```python
from build123d import *

# Parameters (mm, degrees)
SKETCH1_W                   = 58
SKETCH1_H                   = 13
BOSS_EXTRUDE1_DEPTH         = 30
FILLET1_R                   = 2
FILLET2_R                   = 3
M6_TAPPED_HOLE1_D           = 5
M6_TAPPED_HOLE1_DEPTH       = 17
M6_TAPPED_HOLE1_CSINK_D     = 6.05
M6_TAPPED_HOLE1_CSINK_ANGLE = 90
M6_TAPPED_HOLE1_TIP         = 1.502151548
CUT_EXTRUDE1_DEPTH          = 24


with BuildPart() as part:
    # Sketch1 → Boss-Extrude1 (new body)
    with BuildSketch(Plane(origin=(0, 0, 0), x_dir=(1, 0, 0), z_dir=(0, 1, 0))):
        Rectangle(SKETCH1_W, SKETCH1_H)
    extrude(amount=-BOSS_EXTRUDE1_DEPTH)

    # Fillet1
    fillet1_edges = [part.edges().sort_by_distance(p)[0] for p in [
        (29, -15, 6.5),
        (-29, -15, 6.5),
        (-29, -15, -6.5),
        (29, -15, -6.5),
    ]]
    fillet(fillet1_edges, radius=FILLET1_R)

    # Fillet2
    # the kernel refuses this fillet: 3 mm, written as the material it takes off along each edge
    with BuildSketch(Plane(origin=(-34.5, 0, 6.5), x_dir=(0, -1, 0), z_dir=(1, 0, 0))) as fillet2_piece_1:
        with BuildLine():
            CenterArc((FILLET2_R, FILLET2_R), FILLET2_R, 180, 90)
            Line((0, FILLET2_R), (0, 0))
            Line((0, 0), (FILLET2_R, 0))
        make_face()
    extrude(amount=69, mode=Mode.SUBTRACT)

    # M6 Tapped Hole1
    with Locations(Plane(origin=(0, -30, 0), x_dir=(-1, 0, 0), z_dir=(0, -1, 0))):
        with Locations((-21.5, 0), (21.5, 0)):
            CounterSinkHole(M6_TAPPED_HOLE1_D / 2, M6_TAPPED_HOLE1_CSINK_D / 2, depth=M6_TAPPED_HOLE1_DEPTH, counter_sink_angle=M6_TAPPED_HOLE1_CSINK_ANGLE)
            with Locations((0, 0, -(M6_TAPPED_HOLE1_DEPTH + M6_TAPPED_HOLE1_TIP / 2))):  # 118° drill point
                Cone(0, M6_TAPPED_HOLE1_D / 2, M6_TAPPED_HOLE1_TIP, mode=Mode.SUBTRACT)

    # Sketch5 → Cut-Extrude1 (cut, symmetric)
    with BuildSketch(Plane(origin=(0, 0, 0), x_dir=(0, 0, -1), z_dir=(1, 0, 0))):
        Polygon((-6.5, -8), (-6.115988572, -30), (-6.5, -30), align=None)
    extrude(amount=CUT_EXTRUDE1_DEPTH, both=True, mode=Mode.SUBTRACT)


solid = part.part
```
CAD build for the part. Positions are in the model's coordinates, mm. A direction names the side the tool comes from. Give positions to 0.01 mm unless a question says otherwise; leave off trailing zeros. Order: outer loops, then holes, each group sorted by start corner. A loop starts at its lowest first (then second) coordinate and runs counter-clockwise, first axis right, second up. Notation, with made-up numbers: M 57.5,34.5 L 66.5,34.5 A32 ccw 66.5,73.5 Z; hole C 83,20.25 d1. An arc over 180 degrees is marked long. Put each result on its own line as item: value. Start each with the question number.
(1) Drill centre lines: line 1 along X through (y, z) = (-29, 1.5); line 2 along X through (y, z) = (-25, 0.5); line 3 along Z through (x, y) = (21.5, -21.5). Where is each one in solid material? Low to high.
(2) Saw through at B-B, the plane x = 4.5. Write the cut outline in (y, z), then the cut area to 3 significant figures.
(3) Saw through at A-A, the plane y = -27.5. Write the cut outline in (x, z), then the cut area to 3 significant figures.
(4) Saw through at C-C, the plane y = -19. Write the cut outline in (x, z).
(5) Flat gauge pin, fed straight in: pin 1 Ø6.5 at (x, z) = (-21.5, 0) entering from +Y. Where does the tip first touch, or does it go through?
(6) Which spindle directions (+Z, -Z, +X, -X, +Y, -Y) get a long thin tool onto all of the face, cutting with end or side? Do faces 1 (the cylindrical face through (19, -21, 0)), 2 (the flat face through (29, -15, 0)). Say none if no direction does.
(7) Mould opens along Z. For faces 3 (the flat face through (0, 0, -2)), 4 (the flat face through (-2, -6, 6.5)), 5 (the cylindrical face through (-24, -21, 0)) say: +Z half, -Z half, draft (parallel to the pull), parting line (faces both ways), or undercut.
Check result:
1. line 1: x = -29 to -23.5, -19.5 to 19.5, 23.5 to 29
1. line 2: x = -29 to -23.95, -19.05 to 19.05, 23.95 to 29
1. line 3: z = -6.5 to -2.5, 2.5 to 6.26
2. outline: M -30,-6.5 L 0,-6.5 L 0,3.5 A3 ccw -3,6.5 L -8,6.5 L -30,6.12 Z
2. area: 384 mm2
3. outline: M -29,-4.5 A2 ccw -27,-6.5 L 27,-6.5 A2 ccw 29,-4.5 L 29,4.5 A2 ccw 27,6.5 L 24,6.5 L 24,6.16 L -24,6.16 L -24,6.5 L -27,6.5 A2 ccw -29,4.5 Z; hole C -21.5,0 d5; hole C 21.5,0 d5
3. area: 695 mm2
4. outline: M -29,-4.5 A2 ccw -27,-6.5 L 27,-6.5 A2 ccw 29,-4.5 L 29,4.5 A2 ccw 27,6.5 L 24,6.5 L 24,6.31 L -24,6.31 L -24,6.5 L -27,6.5 A2 ccw -29,4.5 Z; hole C -21.5,0 d5; hole C 21.5,0 d5
5. pin 1: stops at y = 0
6. face 1: -Y
6. face 2: +Z, -Z, +X, +Y, -Y
7. face 3: draft
7. face 4: +Z half
7. face 5: undercut
